from build123d import *

# Parameters (mm, degrees)
OBR_T1_ANGLE = 180


with BuildPart() as part:
    # Szkic1 → Obrót1 (revolve)
    with BuildSketch(Plane.XY):
        with BuildLine():
            Line((16.5, 12.5), (1, 12.5))
            ThreePointArc((1, 12.5), (0.292893219, 12.792893219), (0, 13.5))
            Line((0, 13.5), (0, 17.5))
            Line((0, 17.5), (1, 17.5))
            Line((1, 17.5), (1, 15))
            ThreePointArc((1, 15), (1.292893219, 14.292893219), (2, 14))
            Line((2, 14), (16.5, 14))
            Line((16.5, 14), (16.5, 12.5))
        make_face()
    revolve(axis=Axis((0, 0, 0), (1, 0, 0)), revolution_arc=OBR_T1_ANGLE)


solid = part.part
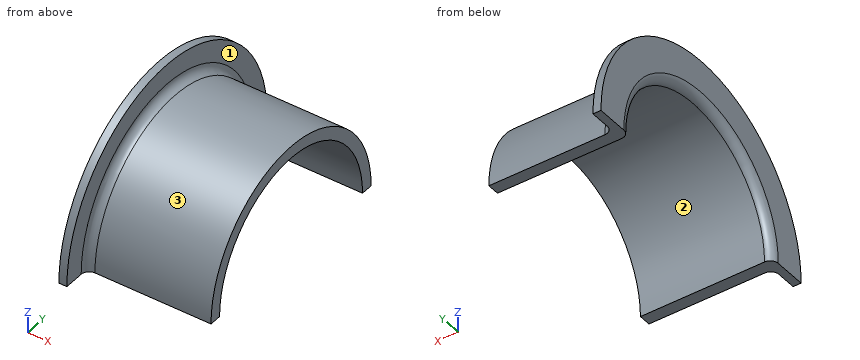
Could you check a few things on this model? Use its own coordinates, in mm. Face numbers are marked on the shaded views. Round coordinates to 2 decimals unless told otherwise and drop trailing zeros. Write each loop counter-clockwise with the first axis right and the second up, starting at its lowest first coordinate (ties: lowest second). Pieces come first, ordered by that corner, then holes. Notation, with made-up numbers: (19.5, -28.5) -> (54.5, -28.5) arc R15 ccw to (54.5, -9.5) -> close; hole circle Ø1 at (83, 40). An arc over 180 degrees is marked (long way). Use a Markdown table: item, result.
1. Please list where these lines run through material, in increasing order: probe 1 along X at (y, z) = (-11.5, 9.5); probe 2 along Z at (x, y) = (13.5, 0); probe 3 along Y at (x, z) = (14.75, 8).
Answer key:
| item | result |
|---|---|
| probe 1 | x = 0 to 1 |
| probe 2 | z = 12.5 to 14 |
| probe 3 | y = -11.49 to -9.6, 9.6 to 11.49 |
2. We'd pull the mould along Y, two halves only. Please class the marked faces 1, 2 and 3: +Y half, -Y half, draft (parallel to the pull), parting line (faces both ways), or undercut.
Answer key:
| item | result |
|---|---|
| face 1 | draft |
| face 2 | undercut |
| face 3 | parting line |
3. If we section it at C-C (z = 16): List the corners of the cut face in (x, y) for me.
Answer key:
| item | result |
|---|---|
| outline | (0, -7.09) -> (1, -7.09) -> (1, 7.09) -> (0, 7.09) -> close |
4. If we section it at A-A (y = 0): List the corners of the cut face in (x, z) for me.
Answer key:
| item | result |
|---|---|
| outline | (0, 13.5) arc R1 ccw to (1, 12.5) -> (16.5, 12.5) -> (16.5, 14) -> (2, 14) arc R1 cw to (1, 15) -> (1, 17.5) -> (0, 17.5) -> close |
5. If we section it at B-B (x = 14.5): List the corners of the cut face in (y, z) for me, then the cut area to 3 significant figures.
Answer key:
| item | result |
|---|---|
| outline | (-14, 0) -> (-12.5, 0) arc R12.5 cw to (12.5, 0) -> (14, 0) arc R14 ccw to start |
| area | 62.4 mm^2 |
6. For pin 1 Ø6 at (x, y) = (12, 8) entering from +Z; pin 2 Ø9 at (y, z) = (3, 10.5) entering from +X; pin 3 Ø1.5 at (x, y) = (2.5, 3.5) entering from +Z; pin 4 Ø4 at (x, y) = (5.5, -8) entering from -Z, each with a flat end and sliding along its axis, tell me the tip position at first contact or that it passes through.
Answer key:
| item | result |
|---|---|
| pin 1 | stops at z = 13.08 |
| pin 2 | stops at x = 16.5 |
| pin 3 | stops at z = 13.73 |
| pin 4 | stops at z = 7.5 |
